Geometry: final body of the model. Coordinates: model frame, mm. Coordinates: 2 decimals unless noted, no trailing zeros. Order: outer loops, then holes, each group sorted by start corner. A loop starts at its lowest first (then second) coordinate and runs counter-clockwise, first axis right, second up. Notation, with made-up numbers: M 12.5,0 L 50.5,0 A29 cw 50.5,36 Z; hole C 54.5,27.5 d5. An arc over 180 degrees is marked long. Use CSV: the item, a comma, the result in double quotes. Start each with the question number.
Q1. Section query A-A, the plane x = 0. Output: boundary loops of the cut face in (y, z), and give its area (3 significant figures).
Q2. Section query B-B, the plane z = 0. Output: boundary loops of the cut face in (x, y).
Q3. First-contact query: P1, Ø12, axis at x = -7.5, y = 276.5, coming from the -Z side; P2, Ø3, axis at x = -48.5, y = 204.5, coming from the +Z side; P3, Ø6, axis at x = 23, y = 204, coming from the -Z side. Flat tips, straight axial feed; report the tip coordinate or a pass-through.
Q4. Ray query, probe 1 along Z at (x, y) = (0, 102); probe 2 along Y at (x, z) = (95, 54); probe 3 along Z at (x, y) = (-71, 323). Return the intervals inside material, ascending.
Q5. Section query D-D, the plane x = -71.25. Output: boundary loops of the cut face in (y, z).
Q6. Section query C-C, the plane y = 44. Output: boundary loops of the cut face in (x, z).
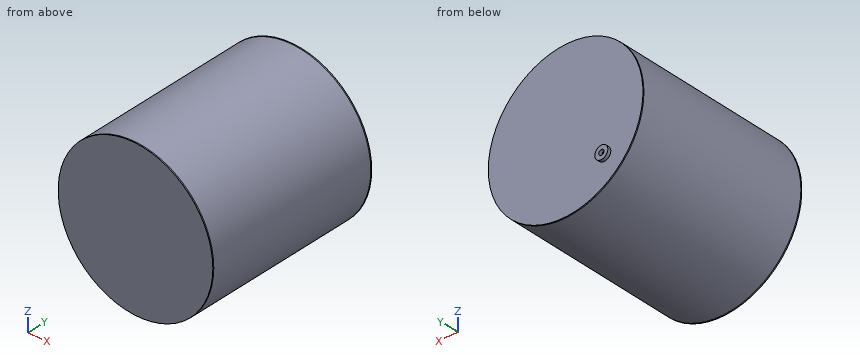
Autodesk Inventor part; units mm, degrees
ref_plane "YZ Plane" through (0, 0, 0) normal (1, 0, 0) x (0, 1, 0)
ref_plane "XZ Plane" through (0, 0, 0) normal (0, 1, 0) x (-1, 0, 0)
ref_plane "XY Plane" through (0, 0, 0) normal (0, 0, 1) x (1, 0, 0)
sketch "Sketch1" plane through (0, 0, 0) normal (0, 1, 0) x (-1, 0, 0)
  circle A0 centre (0, 0) radius 142.5
  circle A1 centre (0, 0) radius 139
  dimension "d0" = 285
  dimension "d1" = 278
extrude "Extrusion1" add sketch "Sketch1" along normal blind 320
sketch "Sketch2" plane through (0, 0, 0) normal (0, -1, 0) x (1, 0, 0)
  circle A0 centre (0, 0) radius 142.5
extrude "Extrusion2" add sketch "Sketch2" along normal blind 2
sketch "Sketch3" plane through (0, 320, 0) normal (0, 1, 0) x (1, 0, 0)
  circle A0 centre (0, 0) radius 142.5
extrude "Extrusion3" add sketch "Sketch3" along normal blind 2
sketch "Sketch4" plane through (0, 322, 0) normal (0, 1, 0) x (1, 0, 0)
  circle A0 centre (0, 0) radius 142.5 construction
  line L0 (0, -142.5) -> (0, 142.5) construction
  line L1 (-142.5, 0) -> (142.5, 0) construction
  line L2 (0, 142.5) -> (-142.5, 0) construction
  line L3 (0, 0) -> (-98.2878, 98.2878) construction
  circle A1 centre (0, 0) radius 139 construction
  circle A2 centre (-71.25, 71.25) radius 7
  dimension "d8" = 14
extrude "Extrusion9" cut sketch "Sketch4" against normal blind 10
sketch "Sketch8" plane through (0, 322, 0) normal (0, 1, 0) x (1, 0, 0)
  circle A0 centre (-71.25, 71.25) radius 7
  circle A1 centre (-71.25, 71.25) radius 4.8
  circle A2 centre (-71.25, 71.25) radius 12
  point P0 (0, 0)
  dimension "d25" = 9.6
  dimension "d26" = 24
extrude "Extrusion10" add sketch "Sketch8" along normal blind 6 contours A0 | A2
properties part number "FermentingTun"
Responses:
1,outline,"M -2,-142.5 L 322,-142.5 L 322,142.5 L -2,142.5 Z; hole M 0,-139 L 320,-139 L 320,139 L 0,139 Z"
1,area,"3,380 mm²"
2,outline,"M -142.5,-2 L 142.5,-2 L 142.5,322 L -142.5,322 Z; hole M -139,0 L 139,0 L 139,320 L -139,320 Z"
3,P1,"stops at z = -142.49"
3,P2,"stops at z = 134.53"
3,P3,"stops at z = -141.09"
4,probe 1,"z = -142.5 to -139, 139 to 142.5"
4,probe 2,"y = -2 to 0, 320 to 322"
4,probe 3,"z = -83.25 to -76.04, -66.46 to -59.25"
5,outline,"M -2,-123.41 L 322,-123.41 L 322,-83.25 L 328,-83.25 L 328,-76.05 L 322,-76.05 L 322,-78.25 L 320,-78.25 L 320,-119.35 L 0,-119.35 L 0,119.35 L 320,119.35 L 320,-64.25 L 322,-64.25 L 322,-66.45 L 328,-66.45 L 328,-59.25 L 322,-59.25 L 322,123.41 L -2,123.41 Z"
6,outline,"C 0,0 d285; hole C 0,0 d278"
